Design review of the part built by this model. Coordinates are the model's own, in mm. A direction names the side the tool comes from. Coordinates: 2 decimals unless noted, no trailing zeros. Loops run counter-clockwise (first coordinate to the right, second up) from the corner with the lowest first, then second, coordinate; pieces in that order, holes last. Notation, with made-up numbers: (8.5, 25) -> (21.5, 25) arc R7 ccw to (21.5, 38) -> close; hole circle Ø6 at (88, -28). An arc over 180 degrees is marked (long way). Use one line per item in the form item = value. Start each with the question number.
1. For pin 1 (1 mm diameter, centred on y = 0, z = -12.5, fed in from +X); pin 2 (1.5 mm diameter, centred on x = 25, y = 4.5, fed in from -Z), all flat-tipped, find the tip position at first contact; note any pin that passes through.
2. Consider section D-D (x = 21.5). State the section outline as (y, z) points, then the cut area to 3 significant figures.
3. Machinability: for faces 4 (the face through (23.535, -2.681, -6.466)), 5 (the face through (23.5, 13, 0)), which of the approach directions +Z, -Z, +X, -X, +Y, -Y give a long, thin tool a straight path to every point of the face, cutting with its end or side? Answer none if there is none.
4. Consider section A-A (y = 0). State the section outline as (x, z) points.
5. Consider section C-C (x = 25.15). State the section outline as (y, z) points.
6. Wall thickness on line 1 (Y direction, x = 24.2, z = 0); line 2 (Y direction, x = 21.75, z = 0.25); line 3 (Z direction, x = 23.6, y = 4.5): over which ranges is each line inside the solid? List them lowest first. Write a range as from..to.
7. The part is to be moulded in two halves that separate along Y. For faces 1 (the face through (26, -6.5, 3.1)), 2 (the face through (23.535, 0.66, 14.985)), 3 (the face through (23.5, -12, 0)), say which applies: released by +Y, released by -Y, zero draft, split by the parting line, or undercut.
from build123d import *

# Parameters (mm, degrees)
SKETCH1_W                      = 5
SKETCH1_H                      = 15
F_14_0_14_DIAMETER_HOLE1_D     = 14
F_2_1_2_1_DIAMETER_HOLE1_D     = 2.1
F_2_1_2_1_DIAMETER_HOLE1_DEPTH = 2.5


with BuildPart() as part:
    # Sketch1 → Revolve1 (revolve)
    with BuildSketch(Plane.XY, mode=Mode.PRIVATE) as revolve1_sk:
        with Locations((23.5, 7.5)):
            Rectangle(SKETCH1_W, SKETCH1_H)
    revolve(revolve1_sk.sketch.rotate(Axis((21, 0, 0), (1, 0, 0)), 270), axis=Axis((21, 0, 0), (1, 0, 0)))

    # Ø14.0 (14) Diameter Hole1 (through all)
    with Locations(Plane.ZY.offset(-21)):
        with Locations((0, 0)):
            Hole(F_14_0_14_DIAMETER_HOLE1_D / 2)

    # Ø2.1 (2.1) Diameter Hole1
    with Locations(Plane(origin=(26, 0, 0), x_dir=(0, 0, -1), z_dir=(1, 0, 0))):
        with Locations((-12.5, 0), (12.5, 0), (0, -12.5), (0, 12.5)):
            Hole(F_2_1_2_1_DIAMETER_HOLE1_D / 2, depth=F_2_1_2_1_DIAMETER_HOLE1_DEPTH)


solid = part.part
Geometry check:
q1.pin_1 = 23.5
q1.pin_2 = -14.52
q2.outline = circle Ø30 at (0, 0); hole circle Ø14 at (0, 0)
q2.area = 553 mm²
q3.face_4 = +X, -X
q3.face_5 = +X
q4.outline = (21, -15) -> (26, -15) -> (26, -13.55) -> (23.5, -13.55) -> (23.5, -11.45) -> (26, -11.45) -> (26, -7) -> (21, -7) -> close; (21, 7) -> (26, 7) -> (26, 11.45) -> (23.5, 11.45) -> (23.5, 13.55) -> (26, 13.55) -> (26, 15) -> (21, 15) -> close
q5.outline = circle Ø30 at (0, 0); hole circle Ø2.1 at (-12.5, 0); hole circle Ø14 at (0, 0); hole circle Ø2.1 at (0, -12.5); hole circle Ø2.1 at (0, 12.5); hole circle Ø2.1 at (12.5, 0)
q6.line_1 = -15..-13.55, -11.45..-7, 7..11.45, 13.55..15
q6.line_2 = -15..-7, 7..15
q6.line_3 = -14.31..-5.36, 5.36..14.31
q7.face_1 = zero draft
q7.face_2 = split by the parting line
q7.face_3 = undercut
